```python
from build123d import *

# Parameters (mm, degrees)
SKETCH1_W           = 107.95
SKETCH1_H           = 12.7
BOSS_EXTRUDE1_DEPTH = 12.7
SKETCH2_R           = 1.778
CUT_EXTRUDE1_DEPTH  = 12.7
SKETCH3_R           = 1.778
CUT_EXTRUDE2_DEPTH  = 12.7
SKETCH4_R           = 1.778
CUT_EXTRUDE3_DEPTH  = 12.7


with BuildPart() as part:
    # Sketch1 → Boss-Extrude1 (new body)
    with BuildSketch(Plane.XY):
        with Locations((53.975, 6.35)):
            Rectangle(SKETCH1_W, SKETCH1_H)
    extrude(amount=BOSS_EXTRUDE1_DEPTH)

    # Sketch2 → Cut-Extrude1 (cut)
    with BuildSketch(Plane(origin=(0, 12.7, 0), x_dir=(1, 0, 0), z_dir=(0, 1, 0))):
        with Locations((101.6, -6.35)):
            Circle(SKETCH2_R)
        with Locations((80.9625, -6.35)):
            Circle(SKETCH2_R)
    extrude(amount=-CUT_EXTRUDE1_DEPTH, mode=Mode.SUBTRACT)

    # Sketch3 → Cut-Extrude2 (cut)
    with BuildSketch(Plane.XZ):
        with Locations((91.28125, 6.35)):
            Circle(SKETCH3_R)
    extrude(amount=-CUT_EXTRUDE2_DEPTH, mode=Mode.SUBTRACT)

    # Sketch4 → Cut-Extrude3 (cut)
    with BuildSketch(Plane(origin=(0, 0, 0), x_dir=(-1, 0, 0), z_dir=(0, 0, -1))):
        with Locations((-12.7, 6.35)):
            Circle(SKETCH4_R)
        with Locations((-50.8, 6.35)):
            Circle(SKETCH4_R)
    extrude(amount=-CUT_EXTRUDE3_DEPTH, mode=Mode.SUBTRACT)


solid = part.part
```
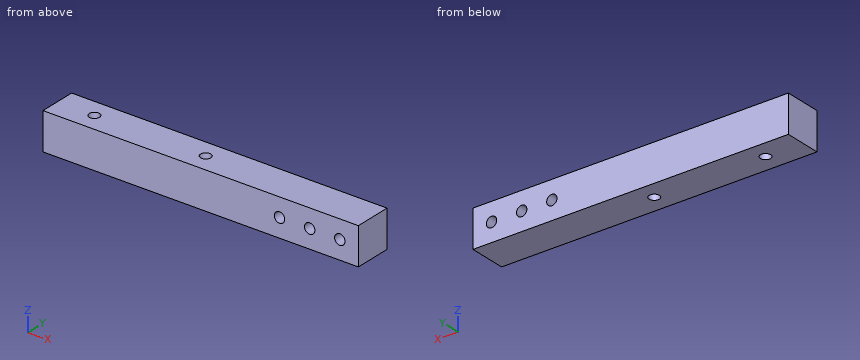
Can you work these out from the model? Positions are in its coordinate system, mm. Coordinates: 2 decimals unless noted, no trailing zeros. Order: outer loops, then holes, each group sorted by start corner. A loop starts at its lowest first (then second) coordinate and runs counter-clockwise, first axis right, second up.
1. I'm going to push a flat-ended pin straight in: pin 1 (5.5 mm diameter, centred on x = 50.8, y = 6.35, fed in from -Z). Where does the tip first touch, or does it pass through?
2. If we section it at D-D (y = 10.5): Please give me the cut outline in (x, z), then the cut area to 3 significant figures.
3. I need wall thicknesses on line 1 (X direction, y = 5.75, z = 1); line 2 (Y direction, x = 12.7, z = 8.25). Which ranges of each line are inside material? Lowest first, please.
4. If we section it at A-A (y = 6.35): Please give me the cut outline in (x, z).
5. If we section it at B-B (z = 6.35): Please give me the cut outline in (x, y).
6. If we section it at C-C (x = 50.8): Please give me the cut outline in (y, z).
Entries:
1. pin 1: stops at z = 0
2. outline: (0, 0) - (107.95, 0) - (107.95, 12.7) - (0, 12.7) - close; hole circle Ø3.56 at (80.96, 6.35); hole circle Ø3.56 at (91.28, 6.35); hole circle Ø3.56 at (101.6, 6.35)
2. area: 1,340 mm2
3. line 1: x = 0 to 11.03, 14.37 to 49.13, 52.47 to 107.95
3. line 2: y = 0 to 4.57, 8.13 to 12.7
4. outline: (0, 0) - (10.92, 0) - (10.92, 12.7) - (0, 12.7) - close; (14.48, 0) - (49.02, 0) - (49.02, 12.7) - (14.48, 12.7) - close; (52.58, 0) - (107.95, 0) - (107.95, 12.7) - (52.58, 12.7) - close; hole circle Ø3.56 at (80.96, 6.35); hole circle Ø3.56 at (91.28, 6.35); hole circle Ø3.56 at (101.6, 6.35)
5. outline: (0, 0) - (79.18, 0) - (79.18, 12.7) - (0, 12.7) - close; (82.74, 0) - (89.5, 0) - (89.5, 12.7) - (82.74, 12.7) - close; (93.06, 0) - (99.82, 0) - (99.82, 12.7) - (93.06, 12.7) - close; (103.38, 0) - (107.95, 0) - (107.95, 12.7) - (103.38, 12.7) - close; hole circle Ø3.56 at (12.7, 6.35); hole circle Ø3.56 at (50.8, 6.35)
6. outline: (0, 0) - (4.57, 0) - (4.57, 12.7) - (0, 12.7) - close; (8.13, 0) - (12.7, 0) - (12.7, 12.7) - (8.13, 12.7) - close
